```python
from build123d import *

# Parameters (mm, degrees)
SKETCH1_R           = 8
SKETCH1_R_2         = 1.6
BOSS_EXTRUDE1_DEPTH = 10
SKETCH2_R           = 3.25
CUT_EXTRUDE1_DEPTH  = 3
SKETCH3_W           = 6.504954041
SKETCH3_H           = 7
BOSS_EXTRUDE2_DEPTH = 1.5
FILLET1_R           = 2


with BuildPart() as part:
    # Sketch1 → Boss-Extrude1 (new body)
    with BuildSketch(Plane.XY):
        with Locations((2, -1)):
            Circle(SKETCH1_R)
        Circle(SKETCH1_R_2, mode=Mode.SUBTRACT)
    extrude(amount=BOSS_EXTRUDE1_DEPTH)

    # Sketch2 → Cut-Extrude1 (cut)
    with BuildSketch(Plane.XY.offset(10)):
        Circle(SKETCH2_R)
    extrude(amount=-CUT_EXTRUDE1_DEPTH, mode=Mode.SUBTRACT)

    # Sketch3 → Cut-Revolve1 (revolve, cut)
    with BuildSketch(Plane(origin=(0, -1, 0), x_dir=(1, 0, 0), z_dir=(0, 1, 0))):
        with Locations((-8.252477021, -5)):
            Rectangle(SKETCH3_W, SKETCH3_H)
    revolve(axis=Axis((2, -1, 0), (0, 0, 1)), mode=Mode.SUBTRACT)

    # Sketch4 → Boss-Extrude2 (add)
    with BuildSketch(Plane.XY):
        with BuildLine():
            Line((-0.911080318, 6.451550938), (12, 11.49549308))
            Line((12, 11.49549308), (12, 0.324258737))
            Line((12, 0.324258737), (8.929423504, -4.997885679))
            ThreePointArc((8.929423504, -4.997885679), (8.06705614, 4.214482697), (-0.911080318, 6.451550938))
        make_face()
    extrude(amount=BOSS_EXTRUDE2_DEPTH)

    # Fillet1
    fillet1_edges = [part.edges().sort_by_distance(p)[0] for p in [
        (12, 11.49549308, 0.75),
    ]]
    fillet(fillet1_edges, radius=FILLET1_R)


solid = part.part
```
Design review of the part built by this model. Coordinates are the model's own, in mm. A direction names the side the tool comes from. Coordinates: 2 decimals unless noted, no trailing zeros. Order: outer loops, then holes, each group sorted by start corner. A loop starts at its lowest first (then second) coordinate and runs counter-clockwise, first axis right, second up. Notation, with made-up numbers: M 87.25,18 L 94.25,18 A30 cw 94.25,53 Z; hole C -26.5,58 d8. An arc over 180 degrees is marked long. Answer as a JSON object with one key per item and string values. Group by question number.
1) Add section C-C, the plane x = 0. Write out the cut boundary in (y, z), then the cut area to 3 significant figures.
2) Wall thickness on L1, parallel to Y at x = -2.75, z = 9.5; L2, parallel to Y at x = 0, z = 7.8; L3, parallel to Z at x = 10.75, y = 2: over which ranges is each line inside the solid? List them lowest first.
3) Add section B-B, the plane z = 4.5. Write out the cut boundary in (x, y).
4) For pin 1 (3 mm diameter, centred on x = 4.5, z = 6, fed in from -Y); pin 2 (5 mm diameter, centred on y = -3, z = 8.5, fed in from +X); pin 3 (3 mm diameter, centred on x = -2.5, z = 2.5, fed in from +Y), all flat-tipped, find the tip position at first contact; note any pin that passes through.
5) Add section A-A, the plane y = -1. Write out the cut boundary in (x, z).
6) Add section D-D, the plane x = 2. Write out the cut boundary in (y, z).
7) Mouldability with a two-part tool opening along X and no side actions: class faces 4 (the flat face through (12, 5, 1)), 5 (the cylindrical face through (3.517, 5.834, 4.951)), 6 (the cylindrical face through (-2.579, -1.978, 8.521)) as pulls with the +X half, pulls with the -X half, needs draft (parallel to the pull), parting line crosses it, or undercut.
8) Tool access review of faces 1 (the flat face through (8.4, 2.3, 1.5)), 2 (the cylindrical face through (5.69, -8.1, 9.24)), 3 (the cylindrical face through (-1.27, -0.97, 3.45)): name each direction out of +Z, -Z, +X, -X, +Y, -Y from which nothing blocks a thin tool from reaching the whole face with its end or side.
Computed values:
{
 "1": {"outline": "M -8.75,0 L -1.6,0 L -1.6,7 L -3.25,7 L -3.25,10 L -8.75,10 L -8.75,8.5 L -7.71,8.5 L -7.71,1.5 L -8.75,1.5 Z; M 1.6,0 L 6.81,0 L 6.81,1.5 L 5.71,1.5 L 5.71,8.5 L 6.75,8.5 L 6.75,10 L 3.25,10 L 3.25,7 L 1.6,7 Z", "area": "98.6 mm^2"},
 "2": {"L1": "y = -7.44 to -1.73, 1.73 to 5.44", "L2": "y = -7.71 to -3.25, 3.25 to 5.71", "L3": "z = 0 to 1.5"},
 "3": {"outline": "C 2,-1 d14; hole C 0,0 d3.2"},
 "4": {"pin 1": "stops at y = -7.93", "pin 2": "stops at x = 10", "pin 3": "stops at y = 6.25"},
 "5": {"outline": "M -6,0 L -1.25,0 L -1.25,7 L -3.09,7 L -3.09,10 L -6,10 L -6,8.5 L -5,8.5 L -5,1.5 L -6,1.5 Z; M 1.25,0 L 11.24,0 L 11.24,1.5 L 9,1.5 L 9,8.5 L 10,8.5 L 10,10 L 3.09,10 L 3.09,7 L 1.25,7 Z"},
 "6": {"outline": "M -9,0 L 7.59,0 L 7.59,1.5 L 6,1.5 L 6,8.5 L 7,8.5 L 7,10 L 2.56,10 L 2.56,7 L -2.56,7 L -2.56,10 L -9,10 L -9,8.5 L -8,8.5 L -8,1.5 L -9,1.5 Z"},
 "7": {"face 4": "pulls with the +X half", "face 5": "parting line crosses it", "face 6": "undercut"},
 "8": {"face 1": "none", "face 2": "+Z", "face 3": "+Z, -Z"}
}
